Read the model definition and answer for the solid it produces. Units are mm, in the model's axes. Give positions to 0.01 mm unless a question says otherwise; leave off trailing zeros. Order: outer loops, then holes, each group sorted by start corner. A loop starts at its lowest first (then second) coordinate and runs counter-clockwise, first axis right, second up. Notation, with made-up numbers: (78, 47.25) - (97, 47.25) arc R11 cw to (97, 51.25) - close; hole circle Ø5 at (-33.5, 22.5). An arc over 180 degrees is marked (long way). Use a Markdown table: item, result. Add a question column.
1. A cutting plane is placed at A-A on z = -5. Determine the outline of the cut face in (x, y) (3 decimals), and give its area (3 significant figures).
2. A cutting plane is placed at C-C on x = 96.52. Determine the outline of the cut face in (y, z) (3 decimals), and give its area (3 significant figures).
3. Consider L1, parallel to X at y = 0.8, z = -5; L2, parallel to Z at x = 96.52, y = 0.65; L3, parallel to Z at x = 27, y = 2.2. Determine where each line is inside the solid, lowest interval first.
4. A cutting plane is placed at D-D on z = -11.75. Determine the outline of the cut face in (x, y) (3 decimals).
5. A cutting plane is placed at B-B on y = 1. Determine the outline of the cut face in (x, z), and give its area (3 significant figures).
6. Flat-ended cylindrical pins translate along their axes: P1, Ø2, axis at x = 29.5, z = -2, coming from the -Y side; P2, Ø1, axis at x = 67.5, y = 2, coming from the -Z side; P3, Ø1, axis at y = 2, z = -12.5, coming from the -X side; P4, Ø2.5, axis at x = 51.6, z = -15, coming from the +Y side. Find the tip coordinate at first contact, or state that the pin passes through.
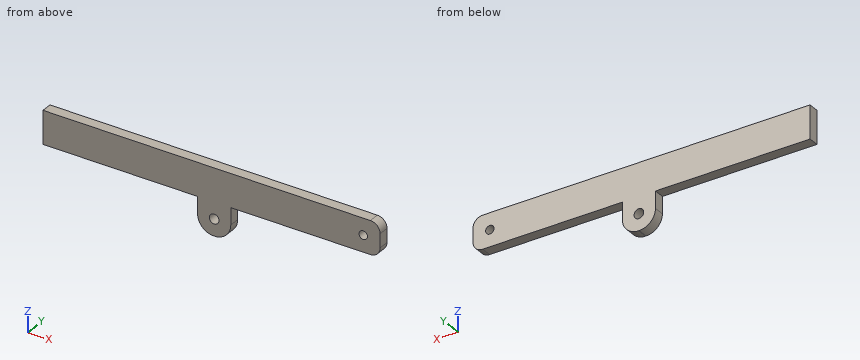
```python
from build123d import *

# Parameters (mm, degrees)
SKETCH1_R           = 1.4605
SKETCH1_R_2         = 1.27
BOSS_EXTRUDE1_DEPTH = 3.175
FILLET1_R           = 2.921


with BuildPart() as part:
    # Sketch1 → Boss-Extrude1 (new body)
    with BuildSketch(Plane(origin=(0, 0, 0), x_dir=(1, 0, 0), z_dir=(0, 1, 0))):
        with BuildLine():
            Line((56.6, 10), (101.6, 10))
            Line((101.6, 10), (101.6, 0))
            Line((101.6, 0), (0, 0))
            Line((0, 0), (0, 10))
            Line((0, 10), (46.6, 10))
            Line((46.6, 10), (46.6, 15.1))
            ThreePointArc((46.6, 15.1), (48.035176772, 18.564823228), (51.5, 20))
            Line((51.5, 20), (51.7, 20))
            ThreePointArc((51.7, 20), (55.164823228, 18.564823228), (56.6, 15.1))
            Line((56.6, 15.1), (56.6, 10))
        make_face()
        with Locations(Location((51.6, 15, 0), (0, 0, 270))):
            Circle(SKETCH1_R, mode=Mode.SUBTRACT)
        with Locations(Location((96.52, 5, 0), (0, 0, 270))):
            Circle(SKETCH1_R_2, mode=Mode.SUBTRACT)
    extrude(amount=BOSS_EXTRUDE1_DEPTH)

    # Fillet1
    fillet1_edges = [part.edges().sort_by_distance(p)[0] for p in [
        (101.6, 1.5875, -10),
        (101.6, 1.5875, 0),
    ]]
    fillet(fillet1_edges, radius=FILLET1_R)


solid = part.part
```
Output values:
| question | item | result |
|---|---|---|
| 1 | outline | (0, 0) - (95.25, 0) - (95.25, 3.175) - (0, 3.175) - close; (97.79, 0) - (101.6, 0) - (101.6, 3.175) - (97.79, 3.175) - close |
| 1 | area | 315 mm² |
| 2 | outline | (0, -10) - (3.175, -10) - (3.175, -6.27) - (0, -6.27) - close; (0, -3.73) - (3.175, -3.73) - (3.175, 0) - (0, 0) - close |
| 2 | area | 23.7 mm² |
| 3 | L1 | 0 to 95.25, 97.79 to 101.6 |
| 3 | L2 | -10 to -6.27, -3.73 to 0 |
| 3 | L3 | -10 to 0 |
| 4 | outline | (46.6, 0) - (56.6, 0) - (56.6, 3.175) - (46.6, 3.175) - close |
| 5 | outline | (0, -10) - (46.6, -10) - (46.6, -15.1) arc R4.9 ccw to (51.5, -20) - (51.7, -20) arc R4.9 ccw to (56.6, -15.1) - (56.6, -10) - (98.68, -10) arc R2.92 ccw to (101.6, -7.08) - (101.6, -2.92) arc R2.92 ccw to (98.68, 0) - (0, 0) - close; hole circle Ø2.92 at (51.6, -15); hole circle Ø2.54 at (96.52, -5) |
| 5 | area | 1,090 mm² |
| 6 | P1 | y = 0 |
| 6 | P2 | z = -10 |
| 6 | P3 | x = 46.6 |
| 6 | P4 | through |
